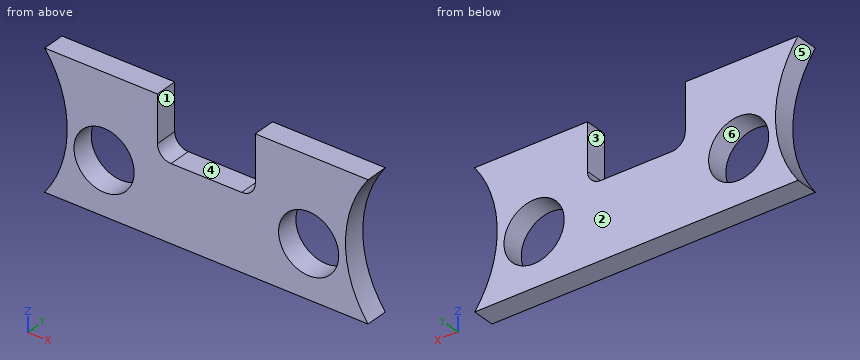
from build123d import *

# Parameters (mm, degrees)
F0_W     = 273.05
F0_H     = 114.3
F1_DEPTH = 19.05
F3_DEPTH = 25.4
F4_R     = 25.4
F5_DEPTH = 25.4


with BuildPart() as f1:
    # F0 (on Front) → F1 (new body)
    with BuildSketch(Plane.XZ):
        with Locations((136.525, 57.15)):
            Rectangle(F0_W, F0_H)
    extrude(amount=F1_DEPTH)

    # F2 (on face) → F3 (cut)
    with BuildSketch(Plane.XZ.offset(19.05)):
        with BuildLine():
            Line((0, 114.3), (0, 0))
            ThreePointArc((0, 0), (19.05, 57.15), (0, 114.3))
        make_face()
        with BuildLine():
            ThreePointArc((273.05, 114.3), (254, 57.15), (273.05, 0))
            Line((273.05, 0), (273.05, 114.3))
        make_face()
    extrude(amount=-F3_DEPTH, mode=Mode.SUBTRACT)

    # F4 (on face) → F5 (cut)
    with BuildSketch(Plane.XZ.offset(19.05)):
        with BuildLine():
            Line((177.8, 114.3), (95.25, 114.3))
            Line((95.25, 114.3), (95.25, 74.93))
            ThreePointArc((95.25, 74.93), (106.68, 86.36), (118.11, 74.93))
            ThreePointArc((118.11, 74.93), (114.762231, 66.847769), (106.68, 63.5))
            Line((106.68, 63.5), (166.37, 63.5))
            ThreePointArc((166.37, 63.5), (158.287769, 83.012231), (177.8, 74.93))
            Line((177.8, 74.93), (177.8, 114.3))
        make_face()
        with Locations((50.163405, 44.45)):
            Circle(F4_R)
        with Locations((222.886595, 44.45)):
            Circle(F4_R)
        with BuildLine():
            ThreePointArc((166.37, 63.5), (174.452231, 66.847769), (177.8, 74.93))
            ThreePointArc((177.8, 74.93), (158.287769, 83.012231), (166.37, 63.5))
        make_face()
        with BuildLine():
            ThreePointArc((118.11, 74.93), (106.68, 86.36), (95.25, 74.93))
            ThreePointArc((95.25, 74.93), (98.597769, 66.847769), (106.68, 63.5))
            ThreePointArc((106.68, 63.5), (114.762231, 66.847769), (118.11, 74.93))
        make_face()
    extrude(amount=-F5_DEPTH, mode=Mode.SUBTRACT)


solid = f1.part
The model under review builds one solid part; all positions refer to its coordinate system, in mm. Face numbers are marked on the shaded views. A direction names the side the tool comes from. Coordinates: 2 decimals unless noted, no trailing zeros. Write each loop counter-clockwise with the first axis right and the second up, starting at its lowest first coordinate (ties: lowest second). Pieces come first, ordered by that corner, then holes. Notation, with made-up numbers: (-37, -17.5) - (15, -17.5) arc R31 cw to (15, 11.5) - close; hole circle Ø6 at (23.5, 57.25). An arc over 180 degrees is marked (long way). Answer as a JSON object with one key per item and string values. Group by question number.
1. Add section C-C (y = -15.5). Give the boundary of the cut face in (x, z), plus the area to 3 significant figures.
2. Add section D-D (z = 44.45). Give the boundary of the cut face in (x, y), plus the area to 3 significant figures.
3. Add section A-A (z = 102). Give the boundary of the cut face in (x, y).
4. To check wall thickness, follow probe 1 along X at (y, z) = (-7.75, 38.5); probe 2 along X at (y, z) = (-3.25, 26.5); probe 3 along Z at (x, y) = (166, -2.5). State the ranges of each line that lie inside material, in increasing order.
5. Machinability: for the marked faces 1 and 2, which of the approach directions +Z, -Z, +X, -X, +Y, -Y give a long, thin tool a straight path to every point of the face, cutting with its end or side? Answer none if there is none.
6. Clearance check with flat-ended pins moving along their axes: pin 1 Ø3 at (y, z) = (-9.5, 73) entering from +X; pin 2 Ø1.5 at (y, z) = (-17, 58) entering from -X; pin 3 Ø9.5 at (x, y) = (132, -8.5) entering from +Z. State where each tip first meets the part, or that it passes through.
7. Mouldability with a two-part tool opening along Z and no side actions: class the marked faces 3, 4, 5 and 6 as pulls with the +Z half, pulls with the -Z half, needs draft (parallel to the pull), parting line crosses it, or undercut.
8. Add section B-B (x = 66). Give the boundary of the cut face in (y, z), plus the area to 3 significant figures.
Findings:
{
 "1": {"outline": "(0, 0) - (273.05, 0) arc R95.25 cw to (273.05, 114.3) - (177.8, 114.3) - (177.8, 74.93) arc R11.43 cw to (166.37, 63.5) - (106.68, 63.5) arc R11.43 cw to (95.25, 74.93) - (95.25, 114.3) - (0, 114.3) arc R95.25 cw to start; hole circle Ø50.8 at (50.16, 44.45); hole circle Ø50.8 at (222.89, 44.45)", "area": "20,100 mm²"},
 "2": {"outline": "(18.2, -19.05) - (24.76, -19.05) - (24.76, 0) - (18.2, 0) - close; (75.56, -19.05) - (197.49, -19.05) - (197.49, 0) - (75.56, 0) - close; (248.29, -19.05) - (254.85, -19.05) - (254.85, 0) - (248.29, 0) - close", "area": "2,570 mm²"},
 "3": {"outline": "(7.83, -19.05) - (95.25, -19.05) - (95.25, 0) - (7.83, 0) - close; (177.8, -19.05) - (265.22, -19.05) - (265.22, 0) - (177.8, 0) - close"},
 "4": {"probe 1": "17.21 to 25.47, 74.86 to 198.19, 247.58 to 255.84", "probe 2": "13.98 to 32.19, 68.13 to 204.92, 240.86 to 259.07", "probe 3": "0 to 63.5"},
 "5": {"face 1": "+Z, +Y, -Y", "face 2": "+Z, -Z, +X, -X, +Y"},
 "6": {"pin 1": "x = 255.59", "pin 2": "x = 19.04", "pin 3": "z = 63.5"},
 "7": {"face 3": "needs draft", "face 4": "pulls with the +Z half", "face 5": "undercut", "face 6": "undercut"},
 "8": {"outline": "(-19.05, 0) - (0, 0) - (0, 24.59) - (-19.05, 24.59) - close; (-19.05, 64.31) - (0, 64.31) - (0, 114.3) - (-19.05, 114.3) - close", "area": "1,420 mm²"}
}
